Source: CAD feature listing. Evaluate the final solid. Frame: model axes, mm. Face numbers are marked on the shaded views. A direction names the side the tool comes from. Round coordinates to 2 decimals unless told otherwise and drop trailing zeros. Loops run counter-clockwise (first coordinate to the right, second up) from the corner with the lowest first, then second, coordinate; pieces in that order, holes last. Notation, with made-up numbers: M 53,-35.5 L 111,-35.5 A23 ccw 111,-18.5 Z; hole C 13.25,65.5 d6. An arc over 180 degrees is marked long. Answer as a JSON object with one key per item and string values.
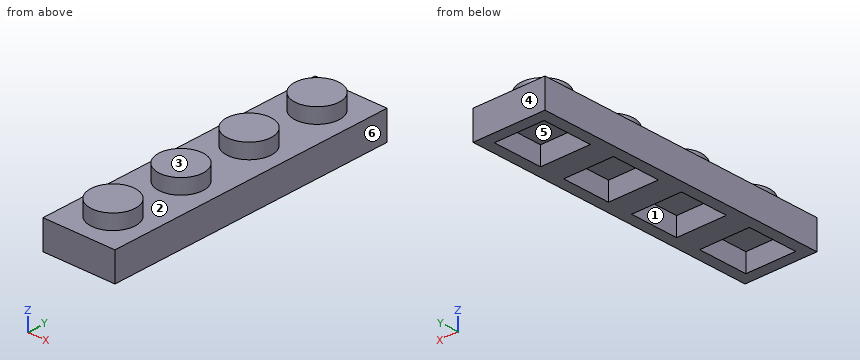
Autodesk Fusion 360 part; units mm, degrees
sketch "Sketch1" plane through (0, 0, 0) normal (0, 0, 1) x (1, 0, 0)
  line L0 (0, 0) -> (7.8, 0)
  line L1 (7.8, 0) -> (7.8, 31.8)
  line L2 (7.8, 31.8) -> (0, 31.8)
  line L3 (0, 31.8) -> (0, 0)
  dimension "d1" = 7.8
  dimension "d2" = 31.8
extrude "Extrude1" add sketch "Sketch1" along normal blind 3.1
sketch "Sketch2" plane through (0, 0, 0) normal (0, 0, -1) x (1, 0, 0)
  line L0 (0, 0) -> (0, -31.8)
  line L1 (0, -31.8) -> (7.8, -31.8)
  line L2 (7.8, -31.8) -> (7.8, 0)
  line L3 (7.8, 0) -> (0, 0)
  line L4 (1.2, -1.2) -> (6.6, -1.2)
  line L5 (6.6, -1.2) -> (6.6, -30.6)
  line L6 (6.6, -30.6) -> (1.2, -30.6)
  line L7 (1.2, -30.6) -> (1.2, -1.2)
  line L8 (-5, -7.95) -> (12, -7.95) construction
  line L9 (-5, -15.9) -> (12, -15.9) construction
  line L10 (-5, -23.85) -> (12, -23.85) construction
  line L11 (1.2, -6.6) -> (6.6, -6.6)
  line L12 (1.2, -9.3) -> (6.6, -9.3)
  line L13 (1.2, -14.55) -> (6.6, -14.55)
  line L14 (1.2, -17.25) -> (6.6, -17.25)
  line L15 (1.2, -22.5) -> (6.6, -22.5)
  line L16 (1.2, -25.2) -> (6.6, -25.2)
  dimension "d5" = 1.2
  dimension "d6" = 1.2
  dimension "d7" = 1.2
  dimension "d8" = 1.2
  dimension "d38" = 7.95
  dimension "d39" = 7.95
  dimension "d40" = 7.95
  dimension "d41" = 1.35
  dimension "d42" = 2.7
  dimension "d43" = 1.35
  dimension "d44" = 2.7
  dimension "d45" = 1.35
  dimension "d46" = 2.7
sketch "Sketch3" plane through (0, 0, 3.1) normal (0, 0, 1) x (-1, 0, 0)
  line L0 (0, -31.8) -> (0, 0)
  line L1 (0, 0) -> (-7.8, 0)
  line L2 (-7.8, 0) -> (-7.8, -31.8)
  line L3 (-7.8, -31.8) -> (0, -31.8)
  circle A0 centre (-3.9, -27.825) radius 2.4
  circle A1 centre (-3.9, -19.875) radius 2.4
  circle A2 centre (-3.9, -11.925) radius 2.4
  circle A3 centre (-3.9, -3.975) radius 2.4
  dimension "d11" = 4.8
  dimension "d12" = 4.8
  dimension "d13" = 4.8
  dimension "d14" = 4.8
  dimension "d15" = 3.9
  dimension "d16" = 7.95
  dimension "d17" = 7.95
  dimension "d18" = 7.95
  dimension "d19" = 3.975
  dimension "d37" = 3.9
extrude "Extrude3" add sketch "Sketch3" along normal blind 1.6 contours A0 | A1 | A2 | A3
extrude "Extrude6" cut sketch "Sketch2" against normal blind 2 contours L4 L5 L7 L11 | L5 L7 L12 L13 | L5 L7 L14 L15 | L5 L6 L7 L16
Item 1: Section B-B on y = 13. Return the cut outline in (x, z), then the cut area to 3 significant figures.
Answer sheet:
{"outline": "M 0,0 L 1.2,0 L 1.2,2 L 6.6,2 L 6.6,0 L 7.8,0 L 7.8,3.1 L 6.05,3.1 L 6.05,4.7 L 1.75,4.7 L 1.75,3.1 L 0,3.1 Z", "area": "20.2 mm²"}
Item 2: Line query: probe 1 along Y at (x, z) = (4.25, 1.2); probe 2 along Y at (x, z) = (4.75, 3.2); probe 3 along X at (y, z) = (21, 1.1). Output: solid intervals per line, ascending. Write a range as from..to.
Answer sheet:
{"probe 1": "y = 0..1.2, 6.6..9.3, 14.55..17.25, 22.5..25.2, 30.6..31.8", "probe 2": "y = 1.73..6.22, 9.68..14.17, 17.63..22.12, 25.58..30.07", "probe 3": "x = 0..1.2, 6.6..7.8"}
Item 3: Contact query for flat-ended pins moving along their axis: pin 1 Ø1 at (x, y) = (4, 16.5) entering from +Z; pin 2 Ø1.6 at (x, y) = (4, 20.5) entering from -Z. Output: stop coordinate, or through.
Answer sheet:
{"pin 1": "stops at z = 3.1", "pin 2": "stops at z = 2"}
Item 4: Pull-direction query (Y, two-part tool) for the marked faces 4, 5 and 6; classes: pulls with the +Y half, pulls with the -Y half, needs draft (parallel to the pull), parting line crosses it, or undercut.
Answer sheet:
{"face 4": "pulls with the +Y half", "face 5": "undercut", "face 6": "needs draft"}
Item 5: Access query for the marked faces 1, 2 and 3. Directions: +Z, -Z, +X, -X, +Y, -Y. A direction counts if a zero-diameter tool reaches every point of the face in a straight line with its end or side. Return the directions, or none.
Answer sheet:
{"face 1": "-Z", "face 2": "+Z", "face 3": "+Z, +X, -X, +Y, -Y"}
Item 6: Section C-C on z = 4. Return the cut outline in (x, y) (3 decimals), then the cut area to 3 significant figures.
Answer sheet:
{"outline": "C 3.9,3.975 d4.8; C 3.9,11.925 d4.8; C 3.9,19.875 d4.8; C 3.9,27.825 d4.8", "area": "72.4 mm²"}
Item 7: Section A-A on z = 1.45. Return the cut outline in (x, y), then the cut area to 3 significant figures.
Answer sheet:
{"outline": "M 0,0 L 7.8,0 L 7.8,31.8 L 0,31.8 Z; hole M 1.2,1.2 L 6.6,1.2 L 6.6,6.6 L 1.2,6.6 Z; hole M 1.2,9.3 L 6.6,9.3 L 6.6,14.55 L 1.2,14.55 Z; hole M 1.2,17.25 L 6.6,17.25 L 6.6,22.5 L 1.2,22.5 Z; hole M 1.2,25.2 L 6.6,25.2 L 6.6,30.6 L 1.2,30.6 Z", "area": "133 mm²"}
